Part model, mm, in its own coordinate system. Face numbers are marked on the shaded views. A direction names the side the tool comes from. Round coordinates to 2 decimals unless told otherwise and drop trailing zeros. Loops run counter-clockwise (first coordinate to the right, second up) from the corner with the lowest first, then second, coordinate; pieces in that order, holes last.
1) Band-saw the part on B-B, the plane x = 22. Write the cut outline in (y, z), then the cut area to 3 significant figures.
2) Drop flat-ended pins along their axis: P1, Ø6, axis at x = 1.5, y = -1.5, coming from the -Z side; P2, Ø5, axis at x = 5.5, z = 2.5, coming from the -Y side; P3, Ø3, axis at x = 19.5, y = 6, coming from the +Z side; P4, Ø1.5, axis at x = 1.5, y = 2, coming from the +Z side. Give the stop position or say it passes through.
3) Probe line 1 (X direction, y = -5.25, z = -3); line 2 (Z direction, x = 7, y = -0.25); line 3 (Y direction, x = -3.5, z = 2.5). List the from-to ranges inside material, lowest first.
4) 3-axis set-ups, long thin cutter, end or side, ignore diameter. For the marked faces 1 and 2: which of +Z, -Z, +X, -X, +Y, -Y reach the whole face in a straight line?
5) Band-saw the part on A-A, the plane x = -2. Write the cut outline in (y, z) (1 decimal).
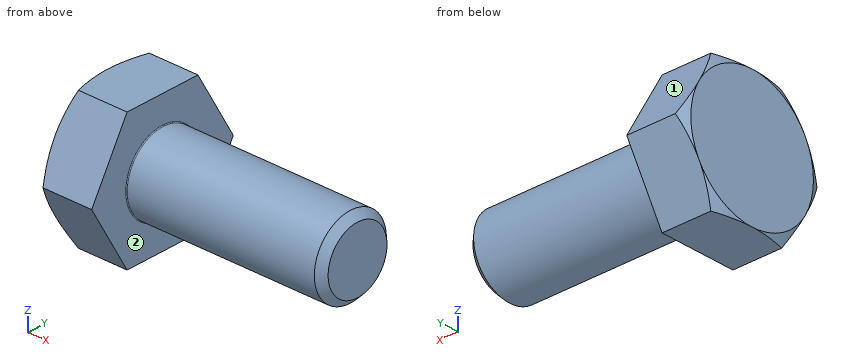
Autodesk Inventor part; units mm, degrees
ref_plane "Work Plane1" through (1.525, 0, 0) normal (0, 0, 1) x (1, 0, 0)
ref_plane "YZ Plane" through (0, 0, 0) normal (1, 0, 0) x (0, 1, 0)
ref_plane "XZ Plane" through (0, 0, 0) normal (0, 1, 0) x (-1, 0, 0)
sketch "Эскиз1" plane through (0, 0, 0) normal (0, 0, 1) x (1, 0, 0)
  line L0 (0, 5) -> (25, 5)
  line L1 (25, 5) -> (25, 0)
  line L2 (25, 0) -> (0, 0)
  line L3 (-5, 0) -> (30, 0)
  line L4 (0, -1) -> (0, 6)
  line L5 (0, 5) -> (0, 0)
  dimension "d2" = 10
  dimension "d59" = 25
revolve "Базовый элемент" add sketch "Эскиз1" angle 360 about axis through (25, 0, 0) along (-1, 0, 0)
sketch "Эскиз2" plane through (0, 0, 0) normal (-1, 0, 0) x (0, 0, 1)
  line L0 (0, 9.815) -> (8.5, 4.9075)
  line L1 (8.5, 4.9075) -> (8.5, -4.9075)
  line L2 (8.5, -4.9075) -> (0, -9.815)
  line L3 (0, -9.815) -> (-8.5, -4.9075)
  line L4 (-8.5, -4.9075) -> (-8.5, 4.9075)
  line L5 (-8.5, 4.9075) -> (0, 9.815)
  line L6 (-11.9, 0) -> (11.9, 0)
  line L7 (0, 13.7409) -> (0, -13.7409)
  point P0 (0, 0)
  point P1 (0, 0)
  dimension "d11" = 17
extrude "С головкой" add sketch "Эскиз2" along normal blind 7
sketch "Эскиз4" plane through (0, 0, 0) normal (0, 0, 1) x (1, 0, 0)
  line L0 (-6.0185, 10.2) -> (-7, 8.5)
  line L1 (-1.1, 0) -> (-0.234, 0)
  line L2 (-8.3532, 0) -> (1.1192, 0)
  line L3 (-7, 10.2) -> (-6.0185, 10.2)
  line L4 (-7, 8.5) -> (-7, 10.2)
  line L5 (0, 12.24) -> (0, -2.04)
  dimension "d65" = 17
  dimension "d67" = 30
  dimension "d68" = 20.4
  dimension "d69" = 7
revolve "Фаска1" cut sketch "Эскиз4" angle 360 about axis through (-1.1, 0, 0) along (1, 0, 0)
thread "Резьба"
chamfer "Фаска2" distance 0.9202 distance2 0.9203 1 edges at (25, -5, 0) measured on face at (25, 1.974, 0.2121)
fillet "Fillet2" radius 0.1 1 edges at (0, -5, 0)
ref_plane "Work Plane1" through (1.525, 0, 0) normal (0, 0, 1) x (1, 0, 0)
equation "\"d2\" = GD"
equation "\"d59\" = NLG"
equation "\"d11\" = SW"
equation "\"d3\" = KOH"
equation "\"d71\" = RR"
equation "\"d15\" = GEL"
equation "\"d6\" = -0.5 * SPD + 0.5 * GD"
equation "\"d65\" = SW"
equation "\"d67\" = ANG1"
equation "\"d68\" = 1.2 * SW"
equation "\"d69\" = KOH"
equation "\"NLG\" = 25"
equation "\"GD\" = 10"
equation "\"KOH\" = 7"
equation "\"GEL\" = 23.5"
equation "\"SW\" = 17"
equation "\"SW0\" = 15.3"
equation "\"SPD\" = NND - 1.2269 * PTC"
equation "\"SD\" = 0"
equation "\"ANG1\" = 30deg"
equation "\"GAL\" = 0.61345 * PTC"
equation "\"GUL\" = 0.61345 * PTC"
equation "\"RR\" = 0.1"
equation "\"RR1\" = 0.1"
equation "\"GD1\" = THREADDIA - 1.2269 * PTC"
equation "\"TOA\" = 30deg"
equation "\"PTC\" = 1.5"
equation "\"E0\" = 1.155 * SW"
properties part number "Болт M10-6gx25 ГОСТ 7805-70" material "Сталь, мягкая"
Reported:
1. outline: circle Ø10 at (0, 0)
1. area: 78.5 mm2
2. P1: stops at z = -8.5
2. P2: stops at y = -5
2. P3: stops at z = 2.18
2. P4: stops at z = 4.84
3. line 1: x = -7 to 0
3. line 2: z = -4.99 to 4.99
3. line 3: y = -8.37 to 8.37
4. face 1: +Z, +X, -X, +Y
4. face 2: +X
5. outline: (-9.8, 0) - (-4.9, -8.5) - (4.9, -8.5) - (9.8, 0) - (4.9, 8.5) - (-4.9, 8.5) - close
